Geometry: final body of the model. Coordinates: model frame, mm. Face numbers are marked on the shaded views. A direction names the side the tool comes from. Round coordinates to 2 decimals unless told otherwise and drop trailing zeros. Loops run counter-clockwise (first coordinate to the right, second up) from the corner with the lowest first, then second, coordinate; pieces in that order, holes last. Notation, with made-up numbers: (-32, 50) - (-16, 50) arc R13 ccw to (-16, 64) - close; hole circle Ø6 at (-33, 76). An arc over 180 degrees is marked (long way). Write item = value, one per line. Start each with the question number.
Item 1: Line query: line 1 (Y direction, x = 64, z = 23); line 2 (Y direction, x = 64.9, z = 23.5); line 3 (Z direction, x = 79, y = 1). Output: solid intervals per line, ascending. Write a range as from..to.
Item 2: Section D-D (x = 70.5). Return loops of the section in (y, z), plus the area to 3 significant figures.
Item 3: Section B-B (z = -23.5). Return loops of the section in (x, y), plus the area to 3 significant figures.
Item 4: Section A-A (x = 83.5). Return loops of the section in (y, z).
Item 5: First-contact query: pin 1 (2 mm diameter, centred on x = 90.5, z = 17.5, fed in from +Y); pin 2 (12 mm diameter, centred on y = 42, z = 4, fed in from -X); pin 3 (6 mm diameter, centred on y = 23, z = 16.5, fed in from +X). Flat tips, straight axial feed; report the tip coordinate or a pass-through.
Item 6: Section C-C (z = 0). Return loops of the section in (x, y), plus the area to 3 significant figures.
Item 7: Access query for the marked faces 1 and 2. Directions: +Z, -Z, +X, -X, +Y, -Y. A direction counts if a zero-diameter tool reaches every point of the face in a straight line with its end or side. Return the directions, or none.
from build123d import *

# Parameters (mm, degrees)
SKETCH1_W                    = 130
SKETCH1_H                    = 65
BASE_FLANGE1_DEPTH           = 3
SKETCH2_R                    = 19.1
SKETCH2_R_2                  = 2.6
CUT_EXTRUDE1_DEPTH           = 135.034510481
CUT_EXTRUDE3_DEPTH           = 135.034510481
SKETCHED_BEND2_OUTLINE_W     = 3
SKETCHED_BEND2_OUTLINE_H     = 65
SKETCHED_BEND2_DEPTH         = 63.020021532
SKETCHED_START               = 63.383443248
SKETCHED_BEND2_2_OUTLINE_W   = 63.979978468
SKETCHED_BEND2_2_OUTLINE_H   = 65
SKETCHED_BEND2_2_OUTLINE_R   = 2.6
SKETCHED_BEND2_2_OUTLINE_R_2 = 19.1
SKETCHED_BEND2_2_DEPTH       = 2.636578284
SKETCHED_START_2             = 63.020021532
SKETCHED_BEND2_3_OUTLINE_W   = 63.979978468
SKETCHED_BEND2_3_OUTLINE_H   = 65
SKETCHED_BEND2_3_OUTLINE_R   = 2.6
SKETCHED_BEND2_3_OUTLINE_R_2 = 19.1
SKETCHED_BEND2_3_DEPTH       = 3.7366
SKETCHED_START_3             = -33
SKETCHED_BEND2_4_DEPTH       = 66
BOSS_EXTRUDE1_DEPTH          = 3
CHAMFER1_SIZE                = 5
CHAMFER2_SIZE                = 0.3


with BuildPart() as part:
    # Base-Flange1: sheet metal written as solids
    # Sketch1 → Base-Flange1 (new body)
    with BuildSketch(Plane(origin=(0, 0, 0), x_dir=(1, 0, 0), z_dir=(0, 1, 0))):
        with Locations((65, 0)):
            Rectangle(SKETCH1_W, SKETCH1_H)
    extrude(amount=-BASE_FLANGE1_DEPTH)

    # Sketch2 → Cut-Extrude1 (cut, through all)
    with BuildSketch(Plane(origin=(0, 0, 0), x_dir=(1, 0, 0), z_dir=(0, 1, 0))):
        with Locations(Location((29, 0, 0), (0, 0, 270))):
            Circle(SKETCH2_R)
        with Locations(Location((5.5, 23.5, 0), (0, 0, 270))):
            Circle(SKETCH2_R_2)
        with Locations(Location((52.5, 23.5, 0), (0, 0, 270))):
            Circle(SKETCH2_R_2)
        with Locations(Location((52.5, -23.5, 0), (0, 0, 270))):
            Circle(SKETCH2_R_2)
        with Locations(Location((5.5, -23.5, 0), (0, 0, 270))):
            Circle(SKETCH2_R_2)
    extrude(amount=-CUT_EXTRUDE1_DEPTH, mode=Mode.SUBTRACT)

    # Sketch4 → Cut-Extrude3 (cut, through all)
    with BuildSketch(Plane(origin=(0, 0, 0), x_dir=(1, 0, 0), z_dir=(0, 1, 0))):
        with BuildLine():
            Line((78, 22.1), (120, 22.1))
            ThreePointArc((120, 22.1), (122.1, 20), (120, 17.9))
            Line((120, 17.9), (78, 17.9))
            ThreePointArc((78, 17.9), (75.9, 20), (78, 22.1))
        make_face()
        with BuildLine():
            Line((78, -17.9), (120, -17.9))
            ThreePointArc((120, -17.9), (122.1, -20), (120, -22.1))
            Line((120, -22.1), (78, -22.1))
            ThreePointArc((78, -22.1), (75.9, -20), (78, -17.9))
        make_face()
    extrude(amount=-CUT_EXTRUDE3_DEPTH, mode=Mode.SUBTRACT)

    # Sketched Bend2: read off the stored shape, not the designer's step
    # Sketched Bend2 outline → Sketched Bend2 (cut)
    with BuildSketch(Plane.YZ):
        with Locations((-1.5, 0)):
            Rectangle(SKETCHED_BEND2_OUTLINE_W, SKETCHED_BEND2_OUTLINE_H)
    extrude(amount=SKETCHED_BEND2_DEPTH, mode=Mode.SUBTRACT)

    # Sketched Bend2 2 outline → Sketched Bend2 2 (add)
    with BuildSketch(Plane.YZ.offset(SKETCHED_START)):
        with Locations((31.989989234, 0)):
            Rectangle(SKETCHED_BEND2_2_OUTLINE_W, SKETCHED_BEND2_2_OUTLINE_H)
        with Locations((11.479978468, -23.5)):
            Circle(SKETCHED_BEND2_2_OUTLINE_R, mode=Mode.SUBTRACT)
        with Locations((58.479978468, -23.5)):
            Circle(SKETCHED_BEND2_2_OUTLINE_R, mode=Mode.SUBTRACT)
        with Locations((11.479978468, 23.5)):
            Circle(SKETCHED_BEND2_2_OUTLINE_R, mode=Mode.SUBTRACT)
        with Locations((34.979978468, 0)):
            Circle(SKETCHED_BEND2_2_OUTLINE_R_2, mode=Mode.SUBTRACT)
        with Locations((58.479978468, 23.5)):
            Circle(SKETCHED_BEND2_2_OUTLINE_R, mode=Mode.SUBTRACT)
    extrude(amount=SKETCHED_BEND2_2_DEPTH)

    # Sketched Bend2 3 outline → Sketched Bend2 3 (add)
    with BuildSketch(Plane.YZ.offset(SKETCHED_START_2)):
        with Locations((31.989989234, 0)):
            Rectangle(SKETCHED_BEND2_3_OUTLINE_W, SKETCHED_BEND2_3_OUTLINE_H)
        with Locations((11.479978468, -23.5)):
            Circle(SKETCHED_BEND2_3_OUTLINE_R, mode=Mode.SUBTRACT)
        with Locations((58.479978468, -23.5)):
            Circle(SKETCHED_BEND2_3_OUTLINE_R, mode=Mode.SUBTRACT)
        with Locations((11.479978468, 23.5)):
            Circle(SKETCHED_BEND2_3_OUTLINE_R, mode=Mode.SUBTRACT)
        with Locations((34.979978468, 0)):
            Circle(SKETCHED_BEND2_3_OUTLINE_R_2, mode=Mode.SUBTRACT)
        with Locations((58.479978468, 23.5)):
            Circle(SKETCHED_BEND2_3_OUTLINE_R, mode=Mode.SUBTRACT)
    extrude(amount=SKETCHED_BEND2_3_DEPTH)

    # Sketched Bend2 4 outline → Sketched Bend2 4 (cut)
    with BuildSketch(Plane.XY.offset(SKETCHED_START_3)):
        with BuildLine():
            Line((66.756621532, 63.979978468), (66.020021532, 63.979978468))
            Line((66.020021532, 63.979978468), (66.020021532, 0.7366))
            ThreePointArc((66.020021532, 0.7366), (66.235766677, 0.215745145), (66.756621532, 0))
            Line((66.756621532, 0), (66.756621532, 63.979978468))
        make_face()
        with BuildLine():
            ThreePointArc((66.756621532, -3), (64.114446333, -1.905575199), (63.020021532, 0.7366))
            Line((63.020021532, 0.7366), (63.020021532, -3))
            Line((63.020021532, -3), (66.756621532, -3))
        make_face()
    extrude(amount=SKETCHED_BEND2_4_DEPTH, mode=Mode.SUBTRACT)

    # Sketch6 → Boss-Extrude1 (add)
    with BuildSketch(Plane.XY.offset(32.5)):
        Polygon((66.020021532, 25), (81.020021532, 0), (68.020021532, 0), (66.020021532, 3.333333333), align=None)
    boss_extrude1 = extrude(amount=-BOSS_EXTRUDE1_DEPTH)

    # Mirror1: Boss-Extrude1 across plane
    add(boss_extrude1.mirror(Plane.XY))

    # Chamfer1
    chamfer1_edges = [part.edges().sort_by_distance(p)[0] for p in [
        (64.520021532, 63.979978468, -32.5),
        (64.520021532, 63.979978468, 32.5),
        (130, -1.5, -32.5),
        (130, -1.5, 32.5),
    ]]
    chamfer(chamfer1_edges, length=CHAMFER1_SIZE)

    # Chamfer2
    chamfer2_edges = [part.edges().sort_by_distance(p)[0] for p in [
        (63.020021532, 15.879978468, 0),
        (66.020021532, 15.879978468, 0),
        (63.020021532, 55.879978468, -23.5),
        (66.020021532, 55.879978468, -23.5),
        (63.020021532, 8.879978468, -23.5),
        (66.020021532, 8.879978468, -23.5),
        (63.020021532, 8.879978468, 23.5),
        (66.020021532, 8.879978468, 23.5),
        (63.020021532, 55.879978468, 23.5),
        (66.020021532, 55.879978468, 23.5),
        (99, 0, -22.1),
        (122.1, 0, -20),
        (99, 0, -17.9),
        (75.9, 0, -20),
        (99, 0, 17.9),
        (122.1, 0, 20),
        (99, 0, 22.1),
        (75.9, 0, 20),
        (75.9, -3, 20),
        (99, -3, 22.1),
        (122.1, -3, 20),
        (99, -3, 17.9),
        (75.9, -3, -20),
        (99, -3, -17.9),
        (122.1, -3, -20),
        (99, -3, -22.1),
    ]]
    chamfer(chamfer2_edges, length=CHAMFER2_SIZE)


solid = part.part
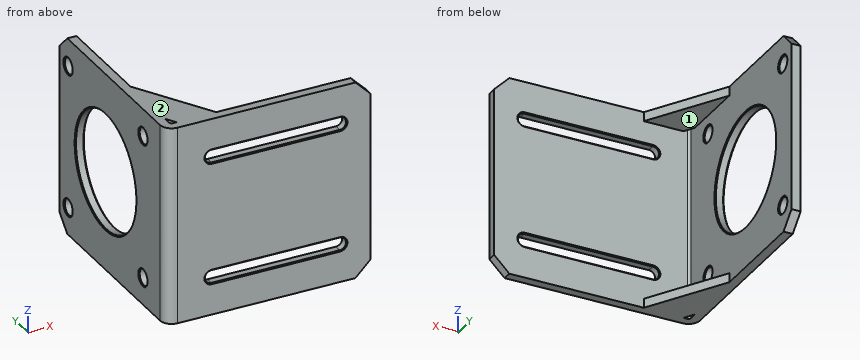
Taken from the geometry:
q1.line_1 = -1.79..8.93, 14.03..55.93, 61.03..63.98
q1.line_2 = -2.51..8.88, 14.08..55.88, 61.08..63.98
q1.line_3 = -32.5..-29.5, 29.5..32.5
q2.outline = (-3, -32.5) - (17.53, -32.5) - (17.53, -29.5) - (0, -29.5) - (0, 29.5) - (17.53, 29.5) - (17.53, 32.5) - (-3, 32.5) - close
q2.area = 300 mm^2
q3.outline = (63.02, 0.74) arc R3.74 ccw to (66.76, -3) - (130, -3) - (130, 0) - (66.76, 0) arc R0.74 cw to (66.02, 0.74) - (66.02, 8.58) - (65.72, 8.88) - (63.32, 8.88) - (63.02, 8.58) - close; (63.02, 14.38) - (63.32, 14.08) - (65.72, 14.08) - (66.02, 14.38) - (66.02, 55.58) - (65.72, 55.88) - (63.32, 55.88) - (63.02, 55.58) - close; (63.02, 61.38) - (63.32, 61.08) - (65.72, 61.08) - (66.02, 61.38) - (66.02, 63.98) - (63.02, 63.98) - close
q3.area = 358 mm^2
q4.outline = (-3, -32.5) - (0, -32.5) - (0, -22.4) - (-0.3, -22.1) - (-2.7, -22.1) - (-3, -22.4) - close; (-3, -17.6) - (-2.7, -17.9) - (-0.3, -17.9) - (0, -17.6) - (0, 17.6) - (-0.3, 17.9) - (-2.7, 17.9) - (-3, 17.6) - close; (-3, 22.4) - (-2.7, 22.1) - (-0.3, 22.1) - (0, 22.4) - (0, 32.5) - (-3, 32.5) - close
q5.pin_1 = 0
q5.pin_2 = through
q5.pin_3 = 66.02
q6.outline = (63.02, 0.74) arc R3.74 ccw to (66.76, -3) - (130, -3) - (130, 0) - (66.76, 0) arc R0.74 cw to (66.02, 0.74) - (66.02, 15.58) - (65.72, 15.88) - (63.32, 15.88) - (63.02, 15.58) - close; (63.02, 54.38) - (63.32, 54.08) - (65.72, 54.08) - (66.02, 54.38) - (66.02, 63.98) - (63.02, 63.98) - close
q6.area = 275 mm^2
q7.face_1 = +X, +Y
q7.face_2 = +Z, +X, -X, +Y, -Y
